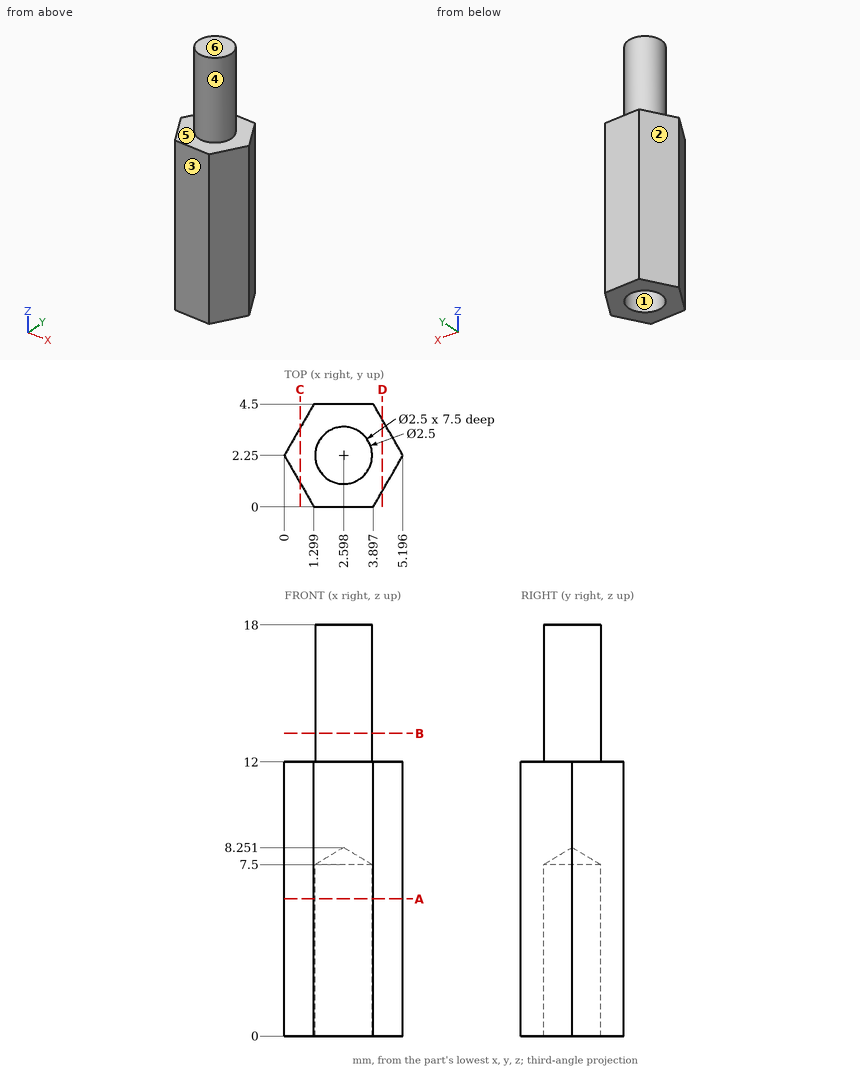
Input: dimensioned drawing with shaded views. Units: mm. Origin: part minimum x, y, z. A direction names the side the tool comes from. Give positions to 0.01 mm unless a question says otherwise; leave off trailing zeros. Loops run counter-clockwise (first coordinate to the right, second up) from the corner with the lowest first, then second, coordinate; pieces in that order, holes last. Notation, with made-up numbers: (79, -17) -> (117, -17) arc R14 ccw to (117, -4) -> close; hole circle Ø6 at (-31, 69.25). An arc over 180 degrees is marked (long way). Use a Markdown table: item, result. Add a question column.
1) Section query C-C, the plane x = 0.7. Return the cut outline in (y, z), then the cut area to 3 significant figures.
2) Section query D-D, the plane x = 4.3. Return the cut outline in (y, z).
3) First-contact query: pin 1 (1.5 mm diameter, centred on x = 3.5, y = 3.5, fed in from -Z). Flat tip, straight axial feed; report the tip coordinate or a pass-through.
4) Pull-direction query (Y, two-part tool) for the marked faces 1, 2, 3 and 4; classes: +Y half, -Y half, draft (parallel to the pull), parting line (faces both ways), or undercut.
5) Section query B-B, the plane z = 13.25. Return the cut outline in (x, y), then the cut area to 3 significant figures.
6) Section query A-A, the plane z = 6. Return the cut outline in (x, y).
7) Reachability of the marked faces 5 and 6 from +Z, -Z, +X, -X, +Y, -Y: full face, straight path, thin tool, end or side. Return the list, or none.
8) Line query: line 1 along Y through (x, z) = (2.7, 7); line 2 along Z through (x, y) = (3.15, 0.85); line 3 along Y through (x, z) = (3.7, 5.5). Output: solid intervals per line, ascending. Write a range as [from, to].
Numbers:
| question | item | result |
|---|---|---|
| 1 | outline | (1.04, 0) -> (3.46, 0) -> (3.46, 12) -> (1.04, 12) -> close |
| 1 | area | 29.1 mm2 |
| 2 | outline | (0.7, 0) -> (3.8, 0) -> (3.8, 12) -> (0.7, 12) -> close |
| 3 | pin 1 | stops at z = 0 |
| 4 | face 1 | undercut |
| 4 | face 2 | +Y half |
| 4 | face 3 | -Y half |
| 4 | face 4 | parting line |
| 5 | outline | circle Ø2.5 at (2.6, 2.25) |
| 5 | area | 4.91 mm2 |
| 6 | outline | (0, 2.25) -> (1.3, 0) -> (3.9, 0) -> (5.2, 2.25) -> (3.9, 4.5) -> (1.3, 4.5) -> close; hole circle Ø2.5 at (2.6, 2.25) |
| 7 | face 5 | +Z |
| 7 | face 6 | +Z, +X, -X, +Y, -Y |
| 8 | line 1 | y = [0, 1], [3.5, 4.5] |
| 8 | line 2 | z = [0, 12] |
| 8 | line 3 | y = [0, 1.66], [2.84, 4.5] |
